Solid Edge part; units mm, degrees
sketch "Sketch1" plane through (0, 0, 0) normal (0, 0, 1) x (1, 0, 0)
  circle A0 centre (0, 0) radius 6
extrude "Protrusion1" add sketch "Sketch1" along normal mid plane 5
hole "hole" at (0, 0, 2.5) direction (0, 0, -1) diameter 5 depth 30 tip angle 118 start chamfer 0.6 start chamfer angle 45 end chamfer 0.6 end chamfer angle 45
sketch "Sketch2" plane through (0, 0, 2.5) normal (0, 0, 1) x (-1, 0, 0)
  line L0 (-25, -4) -> (-4.4721, -4)
  line L1 (-4.4721, -4) -> (-4.4721, 4)
  line L2 (-4.4721, 4) -> (-25, 4)
  line L3 (-25, 4) -> (-25, -4)
  dimension "D1" = 4.4721
extrude "Protrusion2" add sketch "Sketch2" against normal up to vertex (5 mm away)
sketch "Sketch3" plane through (12, 0, -2.5) normal (0, 0, -1) x (1, 0, 0)
  line L0 (13, 4) -> (13, -4)
  line L1 (13, -4) -> (7, -4)
  line L2 (7, -4) -> (7, 4)
  line L3 (7, 4) -> (13, 4)
  dimension "D1" = 7
extrude "ExtrudedProtrusion_4" add sketch "Sketch3" along normal blind 4.25
properties material "Polyethylene, low density"
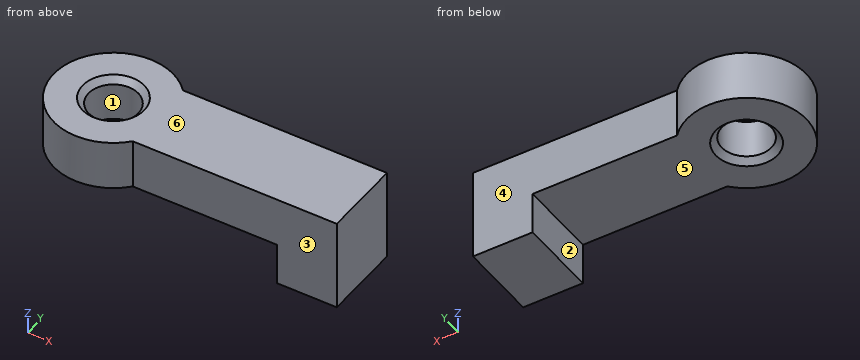
Verification items for the finished model (mm, model axes). Face numbers are marked on the shaded views. A direction names the side the tool comes from. Coordinates: 2 decimals unless noted, no trailing zeros. Order: outer loops, then holes, each group sorted by start corner. A loop starts at its lowest first (then second) coordinate and runs counter-clockwise, first axis right, second up. Notation, with made-up numbers: (10, 81.25) - (66, 81.25) arc R25 cw to (66, 97.25) - close; hole circle Ø5 at (1, 74.25). An arc over 180 degrees is marked (long way). Return JSON: item names as keys, results as strings.
(1) Section check A-A, the plane y = 0. Record the cut outline in (x, z), and give its area (3 significant figures).
Filled sheet:
{"outline": "(-6, -2.5) - (-3.1, -2.5) - (-2.5, -1.9) - (-2.5, 1.9) - (-3.1, 2.5) - (-6, 2.5) - close; (2.5, -1.9) - (3.1, -2.5) - (19, -2.5) - (19, -6.75) - (25, -6.75) - (25, 2.5) - (3.1, 2.5) - (2.5, 1.9) - close", "area": "155 mm^2"}
(2) Access from +Z, -Z, +X, -X, +Y, -Y to the whole of each face (thin tool, end or side, straight path). Record for the marked faces 4, 5 and 6.
Filled sheet:
{"face 4": "+Z, -Z, +X, +Y", "face 5": "-Z, -X, +Y, -Y", "face 6": "+Z, +X, -X, +Y, -Y"}
(3) Section check B-B, the plane x = 0. Record the cut outline in (y, z).
Filled sheet:
{"outline": "(-6, -2.5) - (-3.1, -2.5) - (-2.5, -1.9) - (-2.5, 1.9) - (-3.1, 2.5) - (-6, 2.5) - close; (2.5, -1.9) - (3.1, -2.5) - (6, -2.5) - (6, 2.5) - (3.1, 2.5) - (2.5, 1.9) - close"}
(4) Go/stop test with flat-tipped pins: pin 1 (1 mm diameter, centred on x = 21.5, z = -0.5, fed in from +Y); pin 2 (6 mm diameter, centred on x = 3.5, y = 2.5, fed in from -Z); pin 3 (1 mm diameter, centred on x = 19, z = -3, fed in from -Y). Record where each tip stops, or that it passes through.
Filled sheet:
{"pin 1": "stops at y = 4", "pin 2": "stops at z = -2.5", "pin 3": "stops at y = -4"}
(5) Thickness scan on line 1 along Y through (x, z) = (0, -0.4); line 2 along X through (y, z) = (0, 0); line 3 along X through (y, z) = (3.75, -5.5). Record the ranges inside material, lowest first.
Filled sheet:
{"line 1": "y = -6 to -2.5, 2.5 to 6", "line 2": "x = -6 to -2.5, 2.5 to 25", "line 3": "x = 19 to 25"}
(6) Mould release check, pull along Y, two halves, no side actions. Record for the marked faces 1, 2 and 3: pulls with the +Y half, pulls with the -Y half, needs draft (parallel to the pull), parting line crosses it, or undercut.
Filled sheet:
{"face 1": "undercut", "face 2": "needs draft", "face 3": "pulls with the -Y half"}
(7) Section check D-D, the plane x = 7. Record the cut outline in (y, z).
Filled sheet:
{"outline": "(-4, -2.5) - (4, -2.5) - (4, 2.5) - (-4, 2.5) - close"}
(8) Section check C-C, the plane z = 0.25. Record the cut outline in (x, y), and give its area (3 significant figures).
Filled sheet:
{"outline": "(4.47, -4) - (25, -4) - (25, 4) - (4.47, 4) arc R6 ccw (long way) to start; hole circle Ø5 at (0, 0)", "area": "249 mm^2"}
